Source: CAD feature listing. Evaluate the final solid. Frame: model axes, mm. A direction names the side the tool comes from. Round coordinates to 2 decimals unless told otherwise and drop trailing zeros. Loops run counter-clockwise (first coordinate to the right, second up) from the corner with the lowest first, then second, coordinate; pieces in that order, holes last. Notation, with made-up numbers: M -29,-30 L 16,-30 A22 cw 16,-17 Z; hole C 17.25,-38.75 d1. An arc over 180 degrees is marked long. One line per item, written item: value.
from build123d import *

# Parameters (mm, degrees)
F3_T4_DEPTH  = 67.761612304
F3_S5_R      = 45.861643493
F3_T6_DEPTH  = 37
F3_S7_R      = 45.861643493
F3_T8_DEPTH  = 37
F3_T12_DEPTH = 67.761612304
F3_S13_R     = 45.861643493
F3_T14_DEPTH = 37
F3_S15_R     = 45.861643493
F3_T16_DEPTH = 37
F3_T20_DEPTH = 67.761612304
F3_S21_R     = 45.861643493
F3_T22_DEPTH = 37
F3_S23_R     = 45.861643493
F3_T24_DEPTH = 37


# Not quite as in the source:
# - a fillet or chamfer that OpenCascade refuses, or shapes differently, is made with other operations: its cross-section is extruded or revolved along the edge and cut away or added


with BuildPart() as f2:
    # F2: sweep along a path in F1
    with BuildLine(Plane.XY) as f2_path:
        Line((0, 0), (0, -153.106674552))
        Line((0, -153.106674552), (-257.6704025269, -153.106674552))
        Line((-257.6704025269, -153.106674552), (-257.6704025269, -349.6235013008))
    # F0 (on Front) → F2 (sweep)
    with BuildSketch(Plane.XZ):
        with BuildLine():
            Line((0, 0), (44.372734969, 0))
            add(Edge.make_bspline(
                [(44.372734969, 0), (44.372734969, 22.1863674845), (0, 22.1863674845)],
                knots=[3.1415926536, 3.1415926536, 3.1415926536, 4.7123889804, 4.7123889804, 4.7123889804], degree=2, weights=[1, 0.7071067812, 1]))
            Line((0, 22.1863674845), (0, 0))
        make_face()
        with BuildLine():
            add(Edge.make_bspline(
                [(44.372734969, 0), (44.372734969, 22.1863674845), (0, 22.1863674845)],
                knots=[3.1415926536, 3.1415926536, 3.1415926536, 4.7123889804, 4.7123889804, 4.7123889804], degree=2, weights=[1, 0.7071067812, 1]))
            Line((44.372734969, 0), (51.372734969, 0))
            ThreePointArc((51.372734969, 0), (31.0126987208, 23.9683895846), (0, 29.1863674845))
            Line((0, 29.1863674845), (0, 22.1863674845))
        make_face()
    sweep(path=f2_path.line, transition=Transition.RIGHT)

    # F3: chamfer of 15 on 1 edges, made by hand


with BuildPart() as f3_tool2:
    # F3_s3 → F3_t4 (new body)
    with BuildSketch(Plane.XY):
        Polygon((0, -138.106674552), (-15, -153.106674552), (0, -153.106674552), align=None)
    extrude(amount=F3_T4_DEPTH)

    # F3_s5 → F3_t6 (intersect, symmetric)
    with BuildSketch(Plane.XZ.offset(145.6)):
        with Locations((8.3581917564, -15.9072127065)):
            Circle(F3_S5_R)
    extrude(amount=F3_T6_DEPTH, both=True, mode=Mode.INTERSECT)

    # F3_s7 → F3_t8 (intersect, symmetric)
    with BuildSketch(Plane.YZ.offset(-7.5)):
        with Locations((-161.4648663084, -15.9072127065)):
            Circle(F3_S7_R)
    extrude(amount=F3_T8_DEPTH, both=True, mode=Mode.INTERSECT)


with BuildPart() as f2_1:
    add(f2.part)

    # F3_t1: union F3_tool2
    add(f3_tool2.part)


with BuildPart() as f3_tool10:
    # F3_s11 → F3_t12 (new body)
    with BuildSketch(Plane.XY):
        Polygon((0, -138.106674552), (-15, -153.106674552), (0, -153.106674552), align=None)
    extrude(amount=F3_T12_DEPTH)

    # F3_s13 → F3_t14 (cut, symmetric)
    with BuildSketch(Plane.XZ.offset(145.6)):
        with Locations((8.3581917564, -15.9072127065)):
            Circle(F3_S13_R)
    extrude(amount=F3_T14_DEPTH, both=True, mode=Mode.SUBTRACT)

    # F3_s15 → F3_t16 (intersect, symmetric)
    with BuildSketch(Plane.YZ.offset(-7.5)):
        with Locations((-161.4648663084, -15.9072127065)):
            Circle(F3_S15_R)
    extrude(amount=F3_T16_DEPTH, both=True, mode=Mode.INTERSECT)


with BuildPart() as f2_2:
    add(f2_1.part)

    # F3_t9: union F3_tool10
    add(f3_tool10.part)


with BuildPart() as f3_tool18:
    # F3_s19 → F3_t20 (new body)
    with BuildSketch(Plane.XY):
        Polygon((0, -138.106674552), (-15, -153.106674552), (0, -153.106674552), align=None)
    extrude(amount=F3_T20_DEPTH)

    # F3_s21 → F3_t22 (intersect, symmetric)
    with BuildSketch(Plane.XZ.offset(145.6)):
        with Locations((8.3581917564, -15.9072127065)):
            Circle(F3_S21_R)
    extrude(amount=F3_T22_DEPTH, both=True, mode=Mode.INTERSECT)

    # F3_s23 → F3_t24 (cut, symmetric)
    with BuildSketch(Plane.YZ.offset(-7.5)):
        with Locations((-161.4648663084, -15.9072127065)):
            Circle(F3_S23_R)
    extrude(amount=F3_T24_DEPTH, both=True, mode=Mode.SUBTRACT)


with BuildPart() as f2_3:
    add(f2_2.part)

    # F3_t17: union F3_tool18
    add(f3_tool18.part)


solid = f2_3.part
1. Ray query, line 1 (Z direction, x = -154, y = -172.5); line 2 (Y direction, x = -197, z = 22.75); line 3 (Y direction, x = -238, z = 8.5). Return the intervals inside material, ascending. Write a range as [from, to].
Report:
line 1: z = [0, 28.61]
line 2: y = [-186.14, -153.11]
line 3: y = [-349.62, -153.11]
2. Section query A-A (z = 3.75). Return the cut outline in (x, y).
Report:
outline: M -257.67,-349.62 L -207.88,-349.62 L -207.88,-202.9 L 49.79,-202.9 L 49.79,0 L 0,0 L 0,-138.11 L -15,-153.11 L -257.67,-153.11 Z
3. Pin query (flat end, axial travel): pin 1 (14.5 mm diameter, centred on y = -58, z = 12, fed in from -X); pin 2 (2 mm diameter, centred on y = -158, z = 18, fed in from +X); pin 3 (4 mm diameter, centred on x = -110, z = 22.5, fed in from -Y). Return the tip coordinate at first contact, or that it passes through.
Report:
pin 1: stops at x = 0
pin 2: stops at x = 40.3
pin 3: stops at y = -189.35
4. Section query C-C (x = -57.5). Return the cut outline in (y, z).
Report:
outline: M -204.48,0 L -153.11,0 L -153.11,29.19 A45.86 ccw Z
5. Reachability of faces 1 (the face through (-100.986, -187.177, 22.069)), 2 (the face through (-226.268, -274.576, 23.744)), 3 (the face through (0, -70, 15)), 4 (the face through (-237, -349.624, 12)), 5 (the face through (34.899, -103.671, 21.494)) from +Z, -Z, +X, -X, +Y, -Y: full face, straight path, thin tool, end or side. Return the list, or none.
Report:
face 1: +Z
face 2: +Z, -Y
face 3: +Z, -Z, -X, +Y
face 4: +Z, -Z, +X, -X, -Y
face 5: +Z, +Y
6. Section query D-D (x = -228.5). Return the cut outline in (y, z), and give its area (3 significant figures).
Report:
outline: M -349.62,0 L -153.11,0 L -153.11,29.19 A45.86 ccw -182.28,24.96 L -349.62,24.96 Z
area: 5,010 mm2
7. Section query B-B (y = -108.5). Return the cut outline in (x, z).
Report:
outline: M 0,0 L 51.37,0 A45.86 ccw 0,29.19 Z
